Geometry check sheet. Reference: the model listing, model coordinates, mm. A direction names the side the tool comes from. Coordinates: 2 decimals unless noted, no trailing zeros. Write each loop counter-clockwise with the first axis right and the second up, starting at its lowest first coordinate (ties: lowest second). Pieces come first, ordered by that corner, then holes. Notation, with made-up numbers: M 48,-25.75 L 58,-25.75 A25 cw 58,-12.75 Z; hole C 7.5,43 d5. An arc over 180 degrees is marked long. Write each question's results on one line, items separated by ' | '.
```python
from build123d import *

# Parameters (mm, degrees)
F0_W     = 130
F0_H     = 38.1
F2_DEPTH = 3.5
F1_R     = 11
F1_R_2   = 11.05
F3_DEPTH = 12.5
F4_R     = 4
F4_R_2   = 3.95
F5_DEPTH = 7


with BuildPart() as f2:
    # F0 (on Top) → F2 (new body, symmetric)
    with BuildSketch(Plane.XY):
        with Locations((20, 0)):
            Rectangle(F0_W, F0_H)
    extrude(amount=F2_DEPTH, both=True)

    # F1 (on face) → F3 (cut, symmetric)
    with BuildSketch(Plane.XY):
        Polygon((9.33, -5.4848275573), (9.33, 5.4848275573), (0, 10.9696551146), (-9.5, 5.4848275573), (-9.5, -5.4848275573), (0, -10.9696551146), align=None)
        with Locations((27.3575689644, 0)):
            Circle(F1_R)
        Polygon((-19.5691703558, -5.4848275573), (-19.5691703558, 5.4848275573), (-29.0691703558, 10.9696551146), (-38.5691703558, 5.4848275573), (-38.5691703558, -5.4848275573), (-29.0691703558, -10.9696551146), align=None)
        with Locations((57.105883956, 0)):
            Circle(F1_R_2)
    extrude(amount=F3_DEPTH, both=True, mode=Mode.SUBTRACT)

    # F4 (on face) → F5 (join)
    with BuildSketch(Plane.XY.offset(3.5)):
        with Locations((78, 12.05)):
            Circle(F4_R)
        with Locations((-38, 12.05)):
            Circle(F4_R_2)
    extrude(amount=F5_DEPTH)


solid = f2.part
```
Q1. Depth check by flat-ended pin: P1, Ø1.5, axis at y = 14, z = 6, coming from the +X side; P2, Ø3, axis at x = 63.5, y = -14.5, coming from the +Z side; P3, Ø10, axis at x = 50.5, y = 5, coming from the -Z side. Enter the tip coordinate at first touch or a pass-through.
Geometry check:
P1: stops at x = 81.82 | P2: stops at z = 3.5 | P3: stops at z = -3.5
Q2. Mould release check, pull along Y, two halves, no side actions. Record for faces 1 (the cylindrical face through (67.313, -4.232, 0.049)), 2 (the cylindrical face through (75.05, 14.75, 6.95)), 3 (the flat face through (19, 9, -3.5)): pulls with the +Y half, pulls with the -Y half, needs draft (parallel to the pull), parting line crosses it, or undercut.
Geometry check:
face 1: undercut | face 2: parting line crosses it | face 3: needs draft
Q3. Sectioned sample at A-A on y = 0. Record the cut outline in (x, z), and give its area (3 significant figures).
Geometry check:
outline: M -45,-3.5 L -38.57,-3.5 L -38.57,3.5 L -45,3.5 Z; M -19.57,-3.5 L -9.5,-3.5 L -9.5,3.5 L -19.57,3.5 Z; M 9.33,-3.5 L 16.36,-3.5 L 16.36,3.5 L 9.33,3.5 Z; M 38.36,-3.5 L 46.06,-3.5 L 46.06,3.5 L 38.36,3.5 Z; M 68.16,-3.5 L 85,-3.5 L 85,3.5 L 68.16,3.5 Z | area: 336 mm2
Q4. Sectioned sample at B-B on x = 18. Record the cut outline in (y, z), and give its area (3 significant figures).
Geometry check:
outline: M -19.05,-3.5 L -5.78,-3.5 L -5.78,3.5 L -19.05,3.5 Z; M 5.78,-3.5 L 19.05,-3.5 L 19.05,3.5 L 5.78,3.5 Z | area: 186 mm2
Q5. Scan lines: probe 1 along Z at (x, y) = (70.5, -14); probe 2 along X at (y, z) = (-2.5, 2.75); probe 3 along X at (y, z) = (11.5, 7). Record each from-to range of solid material in increasing order.
Geometry check:
probe 1: z = -3.5 to 3.5 | probe 2: x = -45 to -38.57, -19.57 to -9.5, 9.33 to 16.65, 38.07 to 46.34, 67.87 to 85 | probe 3: x = -41.91 to -34.09, 74.04 to 81.96
Q6. Sectioned sample at D-D on z = 7. Record the cut outline in (x, y).
Geometry check:
outline: C -38,12.05 d7.9; C 78,12.05 d8
Q7. Sectioned sample at C-C on z = 0.75. Record the cut outline in (x, y), and give its area (3 significant figures).
Geometry check:
outline: M -45,-19.05 L 85,-19.05 L 85,19.05 L -45,19.05 Z; hole M -38.57,-5.48 L -29.07,-10.97 L -19.57,-5.48 L -19.57,5.48 L -29.07,10.97 L -38.57,5.48 Z; hole M -9.5,-5.48 L 0,-10.97 L 9.33,-5.48 L 9.33,5.48 L 0,10.97 L -9.5,5.48 Z; hole C 27.36,0 d22; hole C 57.11,0 d22.1 | area: 3,570 mm2
Q8. Access from +Z, -Z, +X, -X, +Y, -Y to the whole of each face (thin tool, end or side, straight path). Record for faces 4 (the cylindrical face through (-36.177, 8.546, 6.951)), 5 (the flat face through (19, 19.05, 0)), 6 (the flat face through (-19.569, 0, 0)).
Geometry check:
face 4: +Z | face 5: +Z, -Z, +X, -X, +Y | face 6: +Z, -Z
